Study the drawing (mm; zero at the part's minimum x, y, z) and answer. A direction names the side the tool comes from. Give positions to 0.01 mm unless a question says otherwise; leave off trailing zeros. Order: outer loops, then holes, each group sorted by start corner. A loop starts at its lowest first (then second) coordinate and runs counter-clockwise, first axis right, second up. Notation, with made-up numbers: (-38.75, 69) - (-27.75, 69) arc R18 cw to (-27.75, 74) - close; hole circle Ø5 at (-1.75, -6.5). An arc over 180 degrees is marked (long way). Write each question's results on one line, items separated by ' | '. Start each with the question number.
Q1. Find section A-A on z = 5. Give the vertices of the cut face in (x, y), and give its area (3 significant figures).
Q2. Find section B-B on x = 10. Give the vertices of the cut face in (y, z).
Q3. Find the intervals of material crossed by line 1 along Y through (x, z) = (27.8, 5); line 2 along X through (y, z) = (4, 2.5); line 3 along Y through (x, z) = (19.25, 9.75), in increasing order. Write a range as from..to.
Q4. For a pull along X with two mould halves and no side action, classify the marked faces 1, 2 and 3 as +X half, -X half, draft (parallel to the pull), parting line (faces both ways), or undercut.
Q5. Find section C-C on x = 27.25. Give the vertices of the cut face in (y, z), and give its area (3 significant figures).
Q6. Find section D-D on z = 8. Give the vertices of the cut face in (x, y).
Q7. A tool of negligible diameter and unlimited length cuts with its end or side. For the marked faces 4 and 5, from which of +Z, -Z, +X, -X, +Y, -Y can it reach the whole face along a straight path? Write none if from no direction.
Q8. Flat-ended cylindrical pins translate along their axes: P1, Ø2.5, axis at y = 3.268, z = 5, coming from the -X side; P2, Ø3, axis at y = 9.5, z = 2.5, coming from the -X side; P3, Ø4, axis at x = 4.5, z = 8, coming from the -Y side. Find the tip coordinate at first contact, or state that the pin passes through.
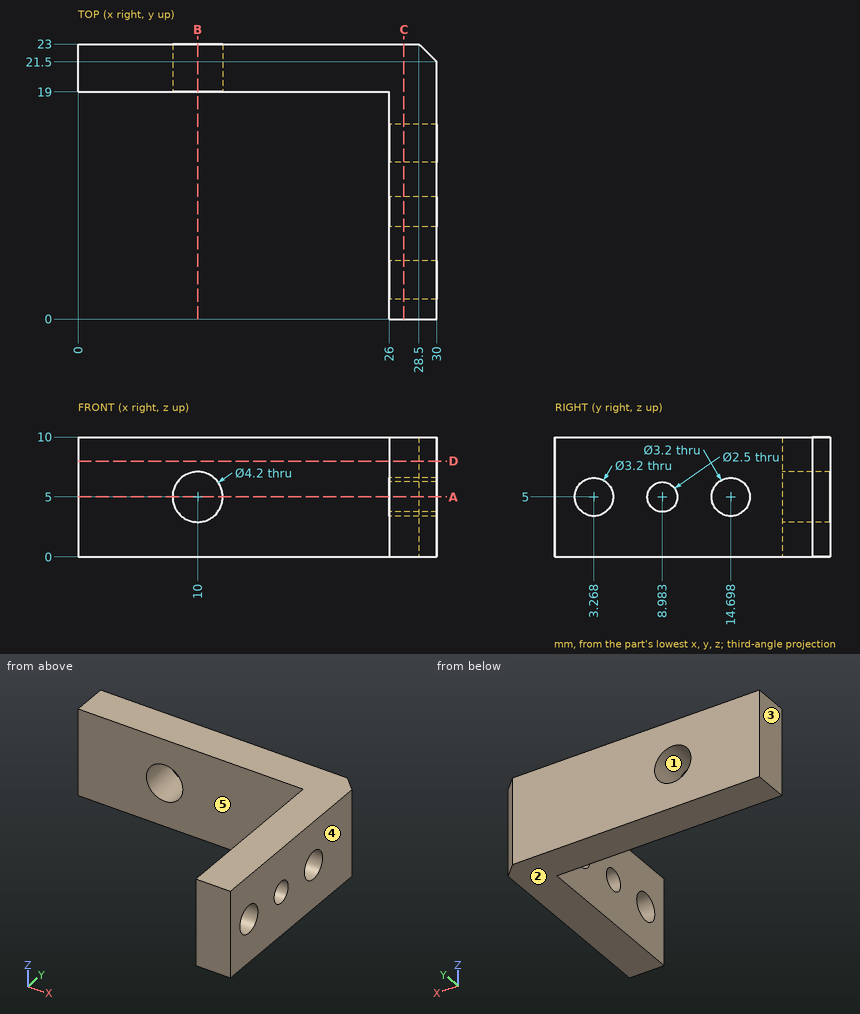
Working result:
1) outline: (0, 19) - (7.9, 19) - (7.9, 23) - (0, 23) - close; (12.1, 19) - (26, 19) - (26, 16.3) - (30, 16.3) - (30, 21.5) - (28.5, 23) - (12.1, 23) - close; (26, 0) - (30, 0) - (30, 1.67) - (26, 1.67) - close; (26, 4.87) - (30, 4.87) - (30, 7.73) - (26, 7.73) - close; (26, 10.23) - (30, 10.23) - (30, 13.1) - (26, 13.1) - close | area: 142 mm²
2) outline: (19, 0) - (23, 0) - (23, 2.9) - (19, 2.9) - close; (19, 7.1) - (23, 7.1) - (23, 10) - (19, 10) - close
3) line 1: 0..1.67, 4.87..7.73, 10.23..13.1, 16.3..23 | line 2: 26..30 | line 3: 19..23
4) face 1: undercut | face 2: draft | face 3: -X half
5) outline: (0, 0) - (23, 0) - (23, 10) - (0, 10) - close; hole circle Ø3.2 at (3.27, 5); hole circle Ø2.5 at (8.98, 5); hole circle Ø3.2 at (14.7, 5) | area: 209 mm²
6) outline: (0, 19) - (26, 19) - (26, 0) - (30, 0) - (30, 21.5) - (28.5, 23) - (0, 23) - close
7) face 4: +Z, -Z, +X, +Y, -Y | face 5: +Z, -Z, -X, -Y
8) P1: through | P2: x = 26 | P3: y = 19
